from build123d import *

# Parameters (mm, degrees)
BOSS_EXTRUDE2_DEPTH = 250
SKETCH5_R           = 6
CUT_EXTRUDE1_DEPTH  = 6
SKETCH6_R           = 3
CUT_EXTRUDE2_DEPTH  = 684.91866463


with BuildPart() as part:
    # Sketch2 → Boss-Extrude2 (new, symmetric)
    with BuildSketch(Plane.XY):
        Polygon((0, 0), (-443.349160121, 0), (-443.349160121, 30), (-43.349160121, 30), (166.872551321, 480.821915028), (220.358608676, 472.5605613), align=None)
    extrude(amount=BOSS_EXTRUDE2_DEPTH, both=True)

    # Sketch5 → Cut-Extrude1 (cut)
    with BuildSketch(Plane(origin=(0, 30, 0), x_dir=(1, 0, 0), z_dir=(0, 1, 0))):
        with Locations(Location((-343.349160121, -235, 0), (0, 0, 270))):
            Circle(SKETCH5_R)
        with Locations(Location((-243.349160121, -235, 0), (0, 0, 270))):
            Circle(SKETCH5_R)
        with Locations(Location((-143.349160121, -235, 0), (0, 0, 270))):
            Circle(SKETCH5_R)
        with Locations(Location((-143.349160121, 235, 0), (0, 0, 90))):
            Circle(SKETCH5_R)
        with Locations(Location((-243.349160121, 235, 0), (0, 0, 90))):
            Circle(SKETCH5_R)
        with Locations(Location((-343.349160121, 235, 0), (0, 0, 90))):
            Circle(SKETCH5_R)
    extrude(amount=-CUT_EXTRUDE1_DEPTH, mode=Mode.SUBTRACT)

    # Sketch6 → Cut-Extrude2 (cut, through all)
    with BuildSketch(Plane(origin=(0, 24, 0), x_dir=(1, 0, 0), z_dir=(0, 1, 0))):
        with Locations(Location((-143.349160121, 235, 0), (0, 0, 270))):
            Circle(SKETCH6_R)
        with Locations(Location((-243.349160121, 235, 0), (0, 0, 270))):
            Circle(SKETCH6_R)
        with Locations(Location((-343.349160121, 235, 0), (0, 0, 270))):
            Circle(SKETCH6_R)
        with Locations(Location((-343.349160121, -235, 0), (0, 0, 270))):
            Circle(SKETCH6_R)
        with Locations(Location((-243.349160121, -235, 0), (0, 0, 270))):
            Circle(SKETCH6_R)
        with Locations(Location((-143.349160121, -235, 0), (0, 0, 270))):
            Circle(SKETCH6_R)
    extrude(amount=-CUT_EXTRUDE2_DEPTH, mode=Mode.SUBTRACT)


solid = part.part
Verification items for the finished model (mm, model axes). A direction names the side the tool comes from. Coordinates: 2 decimals unless noted, no trailing zeros. Loops run counter-clockwise (first coordinate to the right, second up) from the corner with the lowest first, then second, coordinate; pieces in that order, holes last. Notation, with made-up numbers: M 5,-12.5 L 54,-12.5 A29 cw 54,22.5 Z; hole C 40,79.25 d8. An arc over 180 degrees is marked long. One line per item, written item: value.
1. Section check B-B on x = -91.5. Record the cut outline in (y, z), plus the area to 3 significant figures.
Answers follow:
outline: M 0,-250 L 30,-250 L 30,250 L 0,250 Z
area: 15,000 mm^2
2. Set-up check for faces 1 (the flat face through (13, 135, 250)), 2 (the flat face through (-246, 30, 4)): record each of +Z, -Z, +X, -X, +Y, -Y from which the full face is reachable in a straight line by a thin tool's end or side.
Answers follow:
face 1: +Z, +X, -X, +Y, -Y
face 2: +Z, -Z, -X, +Y
3. Section check C-C on y = 90. Record the cut outline in (x, z), plus the area to 3 significant figures.
Answers follow:
outline: M -15.37,-250 L 41.97,-250 L 41.97,250 L -15.37,250 Z
area: 28,700 mm^2
4. Section check A-A on z = -99. Record the cut outline in (x, y), plus the area to 3 significant figures.
Answers follow:
outline: M -443.35,0 L 0,0 L 220.36,472.56 L 166.87,480.82 L -43.35,30 L -443.35,30 Z
area: 39,100 mm^2
5. Material ranges on line 1 along X through (y, z) = (25.4, -235); line 2 along X through (y, z) = (27.25, 235); line 3 along Y through (x, z) = (-206.5, 97), recorded low to high. Write a range as from..to.
Answers follow:
line 1: -443.35..-349.35, -337.35..-249.35, -237.35..-149.35, -137.35..11.84
line 2: -443.35..-349.35, -337.35..-249.35, -237.35..-149.35, -137.35..12.71
line 3: 0..30
6. Gauge pin test, flat ends, axial feed: P1, Ø5, axis at x = -248, z = 199.5, coming from the -Y side; P2, Ø6, axis at x = -244, z = 237, coming from the +Y side; P3, Ø2, axis at x = -21.5, z = -151, coming from the +Y side; P4, Ø1.5, axis at y = 324.5, z = -104, coming from the -X side. Record the tip position at first contact, or that the pin passes through.
Answers follow:
P1: y = 0
P2: y = 24
P3: y = 79
P4: x = 93.63
